Autodesk Inventor part; units mm, degrees
ref_plane "YZ Plane" through (0, 0, 0) normal (1, 0, 0) x (0, 1, 0)
ref_plane "XZ Plane" through (0, 0, 0) normal (0, 1, 0) x (-1, 0, 0)
ref_plane "XY Plane" through (0, 0, 0) normal (0, 0, 1) x (1, 0, 0)
sketch "Sketch1" plane through (0, 0, 0) normal (0, 1, 0) x (-1, 0, 0)
  circle A0 centre (0, 0) radius 19.05
  dimension "d0" = 38.1
extrude "Extrusion1" add sketch "Sketch1" along normal blind 5.08
chamfer "Chamfer1" distance 12.7 distance2 5.08 1 edges at (19.05, 5.08, 0) measured on face at (1.7089, 5.08, -1.4667)
sketch "Sketch2" plane through (0, 5.08, 0) normal (0, 1, 0) x (1, 0, 0)
  circle A0 centre (0, 0) radius 19.05
  dimension "d6" = 38.1
extrude "Extrusion2" add sketch "Sketch2" along normal blind 5.08
chamfer "Chamfer2" distance 12.7 distance2 5.08 1 edges at (-19.05, 5.08, 0) measured on face at (14.5707, 5.08, 2.0262)
sketch "Sketch5" plane through (0, 10.16, 0) normal (0, 1, 0) x (1, 0, 0)
  circle A0 centre (0, 0) radius 2.54
  dimension "d15" = 5.08
extrude "Extrusion4" cut sketch "Sketch5" against normal blind 10.16
properties part number "Pulley V2"
Geometry: final body of the model. Coordinates: model frame, mm. A direction names the side the tool comes from. Give positions to 0.01 mm unless a question says otherwise; leave off trailing zeros. Write each loop counter-clockwise with the first axis right and the second up, starting at its lowest first coordinate (ties: lowest second). Pieces come first, ordered by that corner, then holes.
1. Reachability of faces 1 (the conical face through (1.549, 4.762, 6.975)), 2 (the flat face through (4, 10.16, 0)) from +Z, -Z, +X, -X, +Y, -Y: full face, straight path, thin tool, end or side. Return the list, or none.
2. Draft query along Z for faces 3 (the cylindrical face through (-0.33, 5.15, -2.52)), 4 (the flat face through (-4, 0, 0)). Return one class per face: released by +Z, released by -Z, zero draft, split by the parting line, or undercut.
3. Section query C-C, the plane y = 8.5. Return loops of the section in (x, z).
4. Pin query (flat end, axial travel): P1, Ø1.5, axis at x = 12, y = 6, coming from the -Z side; P2, Ø12, axis at x = 10.5, z = 2, coming from the -Y side. Return the tip coordinate at first contact, or that it passes through.
5. Section query D-D, the plane y = 2.25. Return loops of the section in (x, z), then the cut area to 3 significant figures.
6. Line query: probe 1 along Y at (x, z) = (-2, -16.5); probe 2 along Y at (x, z) = (-15, 10); probe 3 along Z at (x, y) = (0, 7.5). Output: solid intervals per line, ascending.
Computed:
1. face 1: none
1. face 2: +Z, -Z, +X, -X, +Y
2. face 3: undercut
2. face 4: zero draft
3. outline: circle Ø29.8 at (0, 0); hole circle Ø5.08 at (0, 0)
4. P1: passes through
4. P2: stops at y = 0
5. outline: circle Ø26.85 at (0, 0); hole circle Ø5.08 at (0, 0)
5. area: 546 mm2
6. probe 1: y = 0 to 0.97, 9.19 to 10.16
6. probe 2: y = 0 to 0.41, 9.75 to 10.16
6. probe 3: z = -12.4 to -2.54, 2.54 to 12.4
